Solid Edge part; units mm, degrees
sketch "Sketch1" plane through (0, 0, 0) normal (0, 0, 1) x (1, 0, 0)
  line L0 (2.5, 0) -> (2.5, 30)
  line L1 (0, 30) -> (2.5, 30)
  line L2 (0, 0) -> (0, 30)
  line L3 (0, 0) -> (0, -5)
  line L4 (0, -5) -> (4.25, -5)
  line L5 (4.25, -5) -> (4.25, 0)
  line L6 (4.25, 0) -> (2.5, 0)
revolve "RevolvedProtrusion1" add sketch "Sketch1" angle 360 about axis through (0, 0, 0) along (0, 1, 0)
sketch "Sketch2" plane through (0, 0, 0) normal (1, 0, 0) x (0, 1, 0)
  line L0 (-5, 2.7915) -> (-2.5, 2.7915)
  line L1 (-0.8883, 0) -> (-2.5, 2.7915)
  line L2 (-5, 0) -> (-0.8883, 0)
  line L3 (-5, 0) -> (-5, 2.7915)
revolve "RevolvedCutout1" cut sketch "Sketch2" angle 360 about axis through (0, -4.5, 0) along (0, 1, 0)
sketch "Sketch3" plane through (0, -5, 0) normal (0, -1, 0) x (0, 0, 1)
  circle A0 centre (0, 0) radius 2.7915
  line L0 (-2, -1.1547) -> (0, -2.3094)
  line L1 (0, -2.3094) -> (2, -1.1547)
  line L2 (2, -1.1547) -> (2, 1.1547)
  line L3 (2, 1.1547) -> (0, 2.3094)
  line L4 (0, 2.3094) -> (-2, 1.1547)
  line L5 (-2, 1.1547) -> (-2, -1.1547)
extrude "Protrusion1" add sketch "Sketch3" against normal up to next
sketch "Sketch4" plane through (0, 0, 0) normal (0, 0, 1) x (1, 0, 0)
  line L0 (-2.3094, -5) -> (0, -5)
  line L1 (0, -5) -> (0, -4.3812)
  line L2 (0, -4.3812) -> (-2.3094, -5)
revolve "RevolvedCutout2" cut sketch "Sketch4" angle 360 about axis through (0, -4.5, 0) along (0, 1, 0)
fillet "Round1" radius 0.2 1 edges at (0, 0, -2.5)
fillet "Round2" radius 0.425 1 edges at (0, -5, -4.25)
chamfer "倒斜角_2" distance 0.3333 angle 45 1 edges at (0, 30, -2.5)
cosmetic_thread "螺纹_3" thread depth 24
properties part number "N2611-1313" material "铝 1060"
Design review of the part built by this model. Coordinates are the model's own, in mm. A direction names the side the tool comes from. Round coordinates to 2 decimals unless told otherwise and drop trailing zeros. Write each loop counter-clockwise with the first axis right and the second up, starting at its lowest first coordinate (ties: lowest second). Pieces come first, ordered by that corner, then holes. Notation, with made-up numbers: (47, 2.25) - (69, 2.25) arc R22 cw to (69, 12.25) - close; hole circle Ø2 at (83.5, -36.75). An arc over 180 degrees is marked (long way). Return JSON: item names as keys, results as strings. Group by question number.
Item 1: For probe 1 along Z at (x, y) = (-1.5, 19.5); probe 2 along Y at (x, z) = (2, 2.5); probe 3 along X at (y, z) = (3, 0), list the stretches that pass through material, from the lowest coordinate up. Write a range as [from, to].
Item 2: Machinability: for faces 4 (the face through (1.724, -3.542, -1.014)), 5 (the face through (0, 30, 0)), which of the approach directions +Z, -Z, +X, -X, +Y, -Y give a long, thin tool a straight path to every point of the face, cutting with its end or side? Answer none if there is none.
Item 3: The part is to be moulded in two halves that separate along Z. For faces 1 (the face through (0, 0, 3)), 2 (the face through (-0.54, 15.14, 2.44)), 3 (the face through (1.86, -4.96, -1.09)), say which applies: pulls with the +Z half, pulls with the -Z half, needs draft (parallel to the pull), parting line crosses it, or undercut.
Item 4: We need section A-A on y = 7. Write out the cut boundary in (x, z).
Item 5: Insertion check: P1, Ø3, axis at y = 17.5, z = 3, coming from the +X side; P2, Ø1, axis at x = -1.5, y = 2.5, coming from the +Z side; P3, Ø2, axis at x = 2.5, z = -3.5, coming from the +Y side. Each pin has a flat end and moves straight along its axis. Give the tip position at first contact, or say it passes through.
Model answer:
{
 "1": {"probe 1": "z = [-2, 2]", "probe 2": "y = [-5, 0]", "probe 3": "x = [-2.5, 2.5]"},
 "2": {"face 4": "-Y", "face 5": "+Z, -Z, +X, -X, +Y"},
 "3": {"face 1": "needs draft", "face 2": "parting line crosses it", "face 3": "undercut"},
 "4": {"outline": "circle Ø5 at (0, 0)"},
 "5": {"P1": "stops at x = 2", "P2": "stops at z = 2.29", "P3": "stops at y = 0"}
}
